from build123d import *

# Parameters (mm, degrees)
F1_DEPTH = 228.6


with BuildPart() as f1:
    # F0 (on Front) → F1 (new body)
    with BuildSketch(Plane.XZ):
        with BuildLine():
            ThreePointArc((0, 203.2), (-101.6, 101.6), (0, 0))
            Line((0, 0), (0, 63.5))
            ThreePointArc((0, 63.5), (-38.1, 101.6), (0, 139.7))
            Line((0, 139.7), (0, 203.2))
        make_face()
        with BuildLine():
            Line((-2540, 0), (0, 0))
            ThreePointArc((0, 0), (-101.6, 101.6), (0, 203.2))
            Line((0, 203.2), (-2540, 203.2))
            ThreePointArc((-2540, 203.2), (-2468.1579510314, 173.4420489686), (-2438.4, 101.6))
            ThreePointArc((-2438.4, 101.6), (-2468.1579510314, 29.7579510314), (-2540, 0))
        make_face()
        with BuildLine():
            Line((0, 63.5), (0, 0))
            ThreePointArc((0, 0), (71.8420489686, 29.7579510314), (101.6, 101.6))
            ThreePointArc((101.6, 101.6), (71.8420489686, 173.4420489686), (0, 203.2))
            Line((0, 203.2), (0, 139.7))
            ThreePointArc((0, 139.7), (26.9407683632, 128.5407683632), (38.1, 101.6))
            ThreePointArc((38.1, 101.6), (26.9407683632, 74.6592316368), (0, 63.5))
        make_face()
        with BuildLine():
            ThreePointArc((-2540, 203.2), (-2641.6, 101.6), (-2540, 0))
            Line((-2540, 0), (-2540, 63.5))
            ThreePointArc((-2540, 63.5), (-2578.1, 101.6), (-2540, 139.7))
            Line((-2540, 139.7), (-2540, 203.2))
        make_face()
        with BuildLine():
            Line((-2540, 63.5), (-2540, 0))
            ThreePointArc((-2540, 0), (-2468.1579510314, 29.7579510314), (-2438.4, 101.6))
            ThreePointArc((-2438.4, 101.6), (-2468.1579510314, 173.4420489686), (-2540, 203.2))
            Line((-2540, 203.2), (-2540, 139.7))
            ThreePointArc((-2540, 139.7), (-2513.0592316368, 128.5407683632), (-2501.9, 101.6))
            ThreePointArc((-2501.9, 101.6), (-2513.0592316368, 74.6592316368), (-2540, 63.5))
        make_face()
    extrude(amount=F1_DEPTH)


solid = f1.part
The listing builds one solid part. Answer for the finished solid, in the listing's coordinates (mm). Give positions to 0.01 mm unless a question says otherwise; leave off trailing zeros. Write each loop counter-clockwise with the first axis right and the second up, starting at its lowest first coordinate (ties: lowest second). Pieces come first, ordered by that corner, then holes. Notation, with made-up numbers: (7, -16) -> (54, -16) arc R25 cw to (54, 20) -> close; hole circle Ø7 at (71.5, 83.5). An arc over 180 degrees is marked (long way). One line per question, with ' | ' between items. Start each with the question number.
1. Given pin 1 Ø2 at (y, z) = (-193.5, 139.5) entering from -X, flat-ended and moving along its own axis, determine where the tip first touches the part or whether it passes through.
2. Section A-A (y = -98) is taken. Determine the outline of the cut face in (x, z), plus the area to 3 significant figures.
3. For a pull along X with two mould halves and no side action, classify faces 1 (the cylindrical face through (-2578.063, -112.7, 99.925)), 2 (the cylindrical face through (-2641.575, -112.7, 103.834)), 3 (the flat face through (-1252, -113, 203.2)) as pulls with the +X half, pulls with the -X half, needs draft (parallel to the pull), parting line crosses it, or undercut.
4. Find the intervals of material crossed by probe 1 along X at (y, z) = (-128, 101); probe 2 along Z at (x, y) = (-2540, -163); probe 3 along X at (y, z) = (-72.5, 82.5), in increasing order.
Response values:
1) pin 1: x = -2634.66
2) outline: (-2540, 0) -> (0, 0) arc R101.6 ccw to (0, 203.2) -> (-2540, 203.2) arc R101.6 ccw to start; hole circle Ø76.2 at (-2540, 101.6); hole circle Ø76.2 at (0, 101.6) | area: 539,000 mm2
3) face 1: undercut | face 2: pulls with the -X half | face 3: needs draft
4) probe 1: -2641.6 to -2578.1, -2501.9 to -38.1, 38.1 to 101.6 | probe 2: 0 to 63.5, 139.7 to 203.2 | probe 3: -2639.79 to -2572.97, -2507.03 to -32.97, 32.97 to 99.79
